from build123d import *

# Parameters (mm, degrees)
SKETCH1_R           = 38.1
SKETCH1_R_2         = 10.5
BOSS_EXTRUDE1_DEPTH = 3.175
SKETCH6_R           = 17.75000006
CUT_EXTRUDE2_DEPTH  = 1.500000048
SKETCH8_R           = 2.5527
CUT_EXTRUDE3_DEPTH  = 7.35
SKETCH9_R           = 14.09889992
CUT_EXTRUDE4_DEPTH  = 0.4


with BuildPart() as part:
    # Sketch1 → Boss-Extrude1 (new body, symmetric)
    with BuildSketch(Plane.XY):
        Circle(SKETCH1_R)
        Circle(SKETCH1_R_2, mode=Mode.SUBTRACT)
    extrude(amount=BOSS_EXTRUDE1_DEPTH, both=True)

    # Sketch6 → Cut-Extrude2 (cut)
    with BuildSketch(Plane(origin=(0, 0, -3.175), x_dir=(-1, 0, 0), z_dir=(0, 0, -1))):
        Circle(SKETCH6_R)
    extrude(amount=-CUT_EXTRUDE2_DEPTH, mode=Mode.SUBTRACT)

    # Sketch8 → Cut-Extrude3 (cut, through all)
    with BuildSketch(Plane.XY.offset(3.175)):
        with Locations((-28.871121899, 16.66875)):
            Circle(SKETCH8_R)
        with Locations((0, 33.3375)):
            Circle(SKETCH8_R)
        with Locations((28.871121899, 16.66875)):
            Circle(SKETCH8_R)
        with Locations((28.871121899, -16.66875)):
            Circle(SKETCH8_R)
        with Locations((0, -33.3375)):
            Circle(SKETCH8_R)
        with Locations((-28.871121899, -16.66875)):
            Circle(SKETCH8_R)
    extrude(amount=-CUT_EXTRUDE3_DEPTH, mode=Mode.SUBTRACT)

    # Sketch9 → Cut-Extrude4 (cut)
    with BuildSketch(Plane(origin=(0, 0, -1.674999952), x_dir=(-1, 0, 0), z_dir=(0, 0, -1))):
        Circle(SKETCH9_R)
    extrude(amount=-CUT_EXTRUDE4_DEPTH, mode=Mode.SUBTRACT)


solid = part.part
For this review, take the finished solid that the model builds, in its own axes (mm). A direction names the side the tool comes from. Give positions to 0.01 mm unless a question says otherwise; leave off trailing zeros. Loops run counter-clockwise (first coordinate to the right, second up) from the corner with the lowest first, then second, coordinate; pieces in that order, holes last. Notation, with made-up numbers: (-10, 86) -> (12, 86) arc R13 ccw to (12, 109) -> close; hole circle Ø11 at (64.25, -7). An arc over 180 degrees is marked (long way). One line per question, with ' | ' between items.
1) We need section B-B (x = 0). Write out the cut boundary in (y, z) (3 decimals), plus the area to 3 significant figures.
Resolved:
outline: (-38.1, -3.175) -> (-35.89, -3.175) -> (-35.89, 3.175) -> (-38.1, 3.175) -> close; (-30.785, -3.175) -> (-17.75, -3.175) -> (-17.75, -1.675) -> (-14.099, -1.675) -> (-14.099, -1.275) -> (-10.5, -1.275) -> (-10.5, 3.175) -> (-30.785, 3.175) -> close; (10.5, -1.275) -> (14.099, -1.275) -> (14.099, -1.675) -> (17.75, -1.675) -> (17.75, -3.175) -> (30.785, -3.175) -> (30.785, 3.175) -> (10.5, 3.175) -> close; (35.89, -3.175) -> (38.1, -3.175) -> (38.1, 3.175) -> (35.89, 3.175) -> close | area: 261 mm2
2) The part is to be moulded in two halves that separate along X. For faces 3 (the cylindrical face through (-30.235, -23.183, 0.044)), 4 (the flat face through (8, -8, 3.175)), 5 (the cylindrical face through (-13.024, -5.4, -1.478)), say which applies: +X half, -X half, draft (parallel to the pull), parting line (faces both ways), or undercut.
Resolved:
face 3: parting line | face 4: draft | face 5: undercut
3) We need section D-D (y = -12). Write out the cut boundary in (x, z) (3 decimals), plus the area to 3 significant figures.
Resolved:
outline: (-36.161, -3.175) -> (-13.079, -3.175) -> (-13.079, -1.675) -> (-7.401, -1.675) -> (-7.401, -1.275) -> (7.401, -1.275) -> (7.401, -1.675) -> (13.079, -1.675) -> (13.079, -3.175) -> (36.161, -3.175) -> (36.161, 3.175) -> (-36.161, 3.175) -> close | area: 414 mm2
4) For faces 1 (the flat face through (-1, 15, -1.675)), 2 (the cylindrical face through (10, 3.2, 0.9)), list the 3-axis set-ups (+Z, -Z, +X, -X, +Y, -Y) from which the entire face can be reached by the end or side of a thin tool; tool diameter is ignored.
Resolved:
face 1: -Z | face 2: +Z, -Z
5) We need section C-C (z = 2). Write out the cut boundary in (x, y).
Resolved:
outline: circle Ø76.2 at (0, 0); hole circle Ø5.11 at (-28.87, -16.67); hole circle Ø5.11 at (-28.87, 16.67); hole circle Ø21 at (0, 0); hole circle Ø5.11 at (0, -33.34); hole circle Ø5.11 at (0, 33.34); hole circle Ø5.11 at (28.87, -16.67); hole circle Ø5.11 at (28.87, 16.67)
6) To check wall thickness, follow probe 1 along Y at (x, z) = (0, -2.25); probe 2 along Y at (x, z) = (0, -1.55); probe 3 along X at (y, z) = (0.5, -2.5). State the ranges of each line that lie inside material, in increasing order.
Resolved:
probe 1: y = -38.1 to -35.89, -30.78 to -17.75, 17.75 to 30.78, 35.89 to 38.1 | probe 2: y = -38.1 to -35.89, -30.78 to -14.1, 14.1 to 30.78, 35.89 to 38.1 | probe 3: x = -38.1 to -17.74, 17.74 to 38.1
7) Insertion check: pin 1 Ø22.5 at (x, y) = (3, 7) entering from -Z (3 decimals); pin 2 Ø10.5 at (x, y) = (-5.5, 1.5) entering from -Z (3 decimals); pin 3 Ø2 at (y, z) = (1.5, 0.5) entering from -X; pin 4 Ø2 at (x, z) = (-30.5, -2) entering from -Y. Each pin has a flat end and moves straight along its axis. Give the tip position at first contact, or say it passes through.
Resolved:
pin 1: stops at z = -3.175 | pin 2: stops at z = -1.275 | pin 3: stops at x = -38.1 | pin 4: stops at y = -24.11
8) We need section A-A (y = 0). Write out the cut boundary in (x, z) (3 decimals), plus the area to 3 significant figures.
Resolved:
outline: (-38.1, -3.175) -> (-17.75, -3.175) -> (-17.75, -1.675) -> (-14.099, -1.675) -> (-14.099, -1.275) -> (-10.5, -1.275) -> (-10.5, 3.175) -> (-38.1, 3.175) -> close; (10.5, -1.275) -> (14.099, -1.275) -> (14.099, -1.675) -> (17.75, -1.675) -> (17.75, -3.175) -> (38.1, -3.175) -> (38.1, 3.175) -> (10.5, 3.175) -> close | area: 326 mm2
